from build123d import *

# Parameters (mm, degrees)
F0_R     = 3.5
F0_R_2   = 3.175
F0_R_3   = 4.7625
F1_DEPTH = 2


with BuildPart() as f1:
    # F0 (on Top) → F1 (new body)
    with BuildSketch(Plane.XY):
        with BuildLine():
            ThreePointArc((40, 12.5), (38.535534, 16.035534), (35, 17.5))
            Line((35, 17.5), (-35, 17.5))
            ThreePointArc((-35, 17.5), (-38.535534, 16.035534), (-40, 12.5))
            Line((-40, 12.5), (-40, -12.5))
            ThreePointArc((-40, -12.5), (-38.535534, -16.035534), (-35, -17.5))
            Line((-35, -17.5), (35, -17.5))
            ThreePointArc((35, -17.5), (38.535534, -16.035534), (40, -12.5))
            Line((40, -12.5), (40, 12.5))
        make_face()
        with Locations((-25, 0)):
            Circle(F0_R, mode=Mode.SUBTRACT)
        Circle(F0_R_2, mode=Mode.SUBTRACT)
        with Locations((25, 0)):
            Circle(F0_R_3, mode=Mode.SUBTRACT)
    extrude(amount=F1_DEPTH)


solid = f1.part
Can you work these out from the model? Positions are in its coordinate system, mm. Give positions to 0.01 mm unless a question says otherwise; leave off trailing zeros. Loops run counter-clockwise (first coordinate to the right, second up) from the corner with the lowest first, then second, coordinate; pieces in that order, holes last. Notation, with made-up numbers: (25, -27.75) -> (48, -27.75) arc R9 cw to (48, -20.75) -> close; hole circle Ø3 at (86, 6.25). An arc over 180 degrees is marked (long way). Return JSON: item names as keys, results as strings.
Q1. I want a section at C-C, the plane z = 1.65. Count the separate pieces of the cut face and the enclosed holes in it, then the cut area to 3 significant figures.
Checks:
{"separate pieces": "1", "enclosed holes": "3", "area": "2,640 mm2"}
Q2. I need wall thicknesses on probe 1 along Y at (x, z) = (25, 1.6); probe 2 along Y at (x, z) = (0, 0.85) (3 decimals); probe 3 along X at (y, z) = (-2, 1.25). Which ranges of each line are inside material? Lowest first, please.
Checks:
{"probe 1": "y = -17.5 to -4.76, 4.76 to 17.5", "probe 2": "y = -17.5 to -3.175, 3.175 to 17.5", "probe 3": "x = -40 to -27.87, -22.13 to -2.47, 2.47 to 20.68, 29.32 to 40"}
Q3. I want a section at D-D, the plane x = -25. List the corners of the cut face in (y, z) for me, then the cut area to 3 significant figures.
Checks:
{"outline": "(-17.5, 0) -> (-3.5, 0) -> (-3.5, 2) -> (-17.5, 2) -> close; (3.5, 0) -> (17.5, 0) -> (17.5, 2) -> (3.5, 2) -> close", "area": "56.0 mm2"}
Q4. For pin 1 Ø5 at (x, y) = (0, 0) entering from +Z, with a flat end and sliding along its axis, tell me the tip position at first contact or that it passes through.
Checks:
{"pin 1": "passes through"}
Q5. I want a section at B-B, the plane x = 0. List the corners of the cut face in (y, z) for me (3 decimals), then the cut area to 3 significant figures.
Checks:
{"outline": "(-17.5, 0) -> (-3.175, 0) -> (-3.175, 2) -> (-17.5, 2) -> close; (3.175, 0) -> (17.5, 0) -> (17.5, 2) -> (3.175, 2) -> close", "area": "57.3 mm2"}
Q6. We'd pull the mould along Y, two halves only. Please class faces 1 (the face through (-0.69, -3.1, 0.99)), 2 (the face through (0, 17.5, 1)), 3 (the face through (38.5, -16.07, 0.99)): released by +Y, released by -Y, zero draft, split by the parting line, or undercut.
Checks:
{"face 1": "undercut", "face 2": "released by +Y", "face 3": "released by -Y"}
Q7. I want a section at A-A, the plane y = 0. List the corners of the cut face in (x, z) for me (1 decimal), then the cut area to 3 significant figures.
Checks:
{"outline": "(-40, 0) -> (-28.5, 0) -> (-28.5, 2) -> (-40, 2) -> close; (-21.5, 0) -> (-3.2, 0) -> (-3.2, 2) -> (-21.5, 2) -> close; (3.2, 0) -> (20.2, 0) -> (20.2, 2) -> (3.2, 2) -> close; (29.8, 0) -> (40, 0) -> (40, 2) -> (29.8, 2) -> close", "area": "114 mm2"}
